Design review of the part built by this model. Coordinates are the model's own, in mm. Face numbers are marked on the shaded views. Round coordinates to 2 decimals unless told otherwise and drop trailing zeros. Order: outer loops, then holes, each group sorted by start corner. A loop starts at its lowest first (then second) coordinate and runs counter-clockwise, first axis right, second up.
from build123d import *

# Parameters (mm, degrees)
SKETCH1_W           = 12.7
SKETCH1_H           = 38.1
BOSS_EXTRUDE1_DEPTH = 1.524
SKETCH2_W           = 6.604
SKETCH2_H           = 23.876
SKETCH2_W_2         = 5.334
SKETCH2_H_2         = 22.479000001
BOSS_EXTRUDE2_DEPTH = 2.032
CUT_EXTRUDE2_DEPTH  = 0.508
SKETCH6_W           = 6.731
SKETCH6_H           = 8.89
CUT_EXTRUDE3_DEPTH  = 30.669746225
SKETCH7_W           = 6.6675
SKETCH7_H           = 3.302
CUT_EXTRUDE4_DEPTH  = 0.762


with BuildPart() as part:
    # Sketch1 → Boss-Extrude1 (new body)
    with BuildSketch(Plane(origin=(0, 0, 0), x_dir=(1, 0, 0), z_dir=(0, 1, 0))):
        with Locations((1.262648046, -9.464051393)):
            Rectangle(SKETCH1_W, SKETCH1_H)
    extrude(amount=BOSS_EXTRUDE1_DEPTH)

    # Sketch2 → Boss-Extrude2 (add)
    with BuildSketch(Plane.XZ):
        with Locations((1.262648046, 5.019051392)):
            Rectangle(SKETCH2_W, SKETCH2_H)
        with Locations((1.262648046, 5.082551393)):
            Rectangle(SKETCH2_W_2, SKETCH2_H_2, mode=Mode.SUBTRACT)
    extrude(amount=BOSS_EXTRUDE2_DEPTH)

    # Sketch5 → Cut-Extrude2 (cut)
    with BuildSketch(Plane(origin=(0, 1.524, 0), x_dir=(1, 0, 0), z_dir=(0, 1, 0))):
        with BuildLine():
            ThreePointArc((5.390148046, -9.464051393), (0.008623524, -5.531662964), (-2.102851954, -11.853542134))
            Line((-2.102851954, -11.853542133), (4.628148046, -11.853542133))
            ThreePointArc((4.628148046, -11.853542133), (5.195036474, -10.718075914), (5.390148046, -9.464051393))
        make_face()
        with BuildLine():
            Line((4.628148046, -11.853542133), (-2.102851954, -11.853542133))
            ThreePointArc((-2.102851954, -11.853542134), (1.262648046, -13.591551393), (4.628148046, -11.853542133))
        make_face()
        with BuildLine():
            ThreePointArc((4.628148046, -11.853542133), (1.262648046, -13.591551393), (-2.102851954, -11.853542134))
            Line((-2.102851954, -11.853542133), (-2.102851954, -28.514051393))
            Line((-2.102851954, -28.514051393), (4.628148046, -28.514051393))
            Line((4.628148046, -28.514051393), (4.628148046, -11.853542133))
        make_face()
    extrude(amount=-CUT_EXTRUDE2_DEPTH, mode=Mode.SUBTRACT)

    # Sketch6 → Cut-Extrude3 (cut, through all)
    with BuildSketch(Plane(origin=(0, 1.016, 0), x_dir=(1, 0, 0), z_dir=(0, 1, 0))):
        with Locations((1.262648046, -24.069051393)):
            Rectangle(SKETCH6_W, SKETCH6_H)
    extrude(amount=-CUT_EXTRUDE3_DEPTH, mode=Mode.SUBTRACT)

    # Sketch7 → Cut-Extrude4 (cut)
    with BuildSketch(Plane(origin=(0, 1.016, 0), x_dir=(1, 0, 0), z_dir=(0, 1, 0))):
        with Locations((1.294398046, -17.973051393)):
            Rectangle(SKETCH7_W, SKETCH7_H)
    extrude(amount=-CUT_EXTRUDE4_DEPTH, mode=Mode.SUBTRACT)


solid = part.part
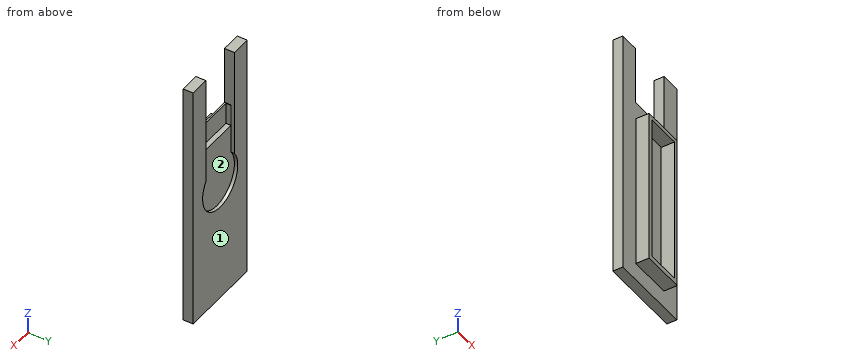
1) To check wall thickness, follow line 1 along Z through (x, y) = (2, -0.4); line 2 along X through (y, z) = (1.15, 20); line 3 along X through (y, z) = (-0.7, -1.5). State the ranges of each line that lie inside material, in increasing order.
Results:
line 1: z = -6.92 to -6.16, 16.32 to 16.96
line 2: x = -5.09 to -2.1, 4.63 to 7.61
line 3: x = -2.04 to -1.4, 3.93 to 4.56
2) Clearance check with flat-ended pins moving along their axes: P1, Ø1.6, axis at x = 1, z = 2, coming from the -Y side; P2, Ø0.8, axis at x = 1.5, y = 0.5, coming from the +Z side; P3, Ø2, axis at x = 1.5, z = 10, coming from the +Y side. State where each tip first meets the part, or that it passes through.
Results:
P1: stops at y = 0
P2: stops at z = 19.62
P3: stops at y = 1.02
3) Take a section at C-C on z = 5. Give the boundary of the cut face in (x, y).
Results:
outline: (-5.09, 0) - (-2.04, 0) - (-2.04, -2.03) - (-1.4, -2.03) - (-1.4, 0) - (3.93, 0) - (3.93, -2.03) - (4.56, -2.03) - (4.56, 0) - (7.61, 0) - (7.61, 1.52) - (-5.09, 1.52) - close
4) The part is to be moulded in two halves that separate along X. For the marked faces 1 and 2, say which applies: released by +X, released by -X, zero draft, split by the parting line, or undercut.
Results:
face 1: zero draft
face 2: undercut
5) Take a section at B-B on z = 24. Give the boundary of the cut face in (x, y), plus the area to 3 significant figures.
Results:
outline: (-5.09, 0) - (-2.1, 0) - (-2.1, 1.52) - (-5.09, 1.52) - close; (4.63, 0) - (7.61, 0) - (7.61, 1.52) - (4.63, 1.52) - close
area: 9.10 mm2
6) Take a section at A-A on y = -1.1. Give the boundary of the cut face in (x, z).
Results:
outline: (-2.04, -6.92) - (4.56, -6.92) - (4.56, 16.96) - (-2.04, 16.96) - close; hole (-1.4, -6.16) - (3.93, -6.16) - (3.93, 16.32) - (-1.4, 16.32) - close
7) Take a section at D-D on x = 3.5. Give the boundary of the cut face in (y, z).
Results:
outline: (-2.03, -6.92) - (0, -6.92) - (0, -9.59) - (1.52, -9.59) - (1.52, 6) - (1.02, 6) - (1.02, 16.32) - (0.25, 16.32) - (0.25, 19.62) - (0, 19.62) - (0, 16.96) - (-2.03, 16.96) - (-2.03, 16.32) - (0, 16.32) - (0, -6.16) - (-2.03, -6.16) - close
